Build history of the part. All positions in model axes, mm. A direction names the side the tool comes from. Give positions to 0.01 mm unless a question says otherwise; leave off trailing zeros. Order: outer loops, then holes, each group sorted by start corner. A loop starts at its lowest first (then second) coordinate and runs counter-clockwise, first axis right, second up. Notation, with made-up numbers: (73.5, -13) - (125.5, -13) arc R16 cw to (125.5, 4) - close; hole circle Ø7 at (72.5, -7.75). An arc over 180 degrees is marked (long way). Answer in a Markdown table with one row per item.
```python
from build123d import *

# Parameters (mm, degrees)
SKETCH1_R           = 0.75
SKETCH1_R_2         = 3.75
BOSS_EXTRUDE1_DEPTH = 3
SKETCH2_W           = 3
SKETCH2_H           = 20
BOSS_EXTRUDE2_DEPTH = 52.5
FILLET5_R           = 10


with BuildPart() as part:
    # Sketch1 → Boss-Extrude1 (new body)
    with BuildSketch(Plane.XY):
        Polygon((0, 0), (-10, 0), (-10, 35), (0, 35), (10, 35), (10, 0), align=None)
        with Locations((-5, 31.95)):
            Circle(SKETCH1_R, mode=Mode.SUBTRACT)
        with Locations((-5, 3.05)):
            Circle(SKETCH1_R, mode=Mode.SUBTRACT)
        with Locations((-5, 17.5)):
            Circle(SKETCH1_R_2, mode=Mode.SUBTRACT)
    extrude(amount=BOSS_EXTRUDE1_DEPTH)

    # Sketch2 → Boss-Extrude2 (add)
    with BuildSketch(Plane(origin=(0, 35, 0), x_dir=(1, 0, 0), z_dir=(0, 1, 0))):
        with Locations((8.5, -10)):
            Rectangle(SKETCH2_W, SKETCH2_H)
    extrude(amount=BOSS_EXTRUDE2_DEPTH)

    # Fillet5
    fillet5_edges = [part.edges().sort_by_distance(p)[0] for p in [
        (8.5, 35, 3),
    ]]
    fillet(fillet5_edges, radius=FILLET5_R)


solid = part.part
```
1. Cut at C-C on y = 3.05. Write the cut outline in (x, z).
Check result:
| item | result |
|---|---|
| outline | (-10, 0) - (-5.75, 0) - (-5.75, 3) - (-10, 3) - close; (-4.25, 0) - (10, 0) - (10, 3) - (-4.25, 3) - close |
2. Two-plate mould, pull along Y, no slides. Class faces 4 (the face through (8, 61, 20)), 5 (the face through (8.48, 31.99, 5.85)), 6 (the face through (-5.098, 32.694, 1.479)): +Y half, -Y half, draft (parallel to the pull), parting line (faces both ways), or undercut.
Check result:
| item | result |
|---|---|
| face 4 | draft |
| face 5 | -Y half |
| face 6 | undercut |
3. Probe line 1 (Y direction, x = -5, z = 2.3); line 2 (Z direction, x = 0, y = 34.5); line 3 (X direction, y = 49, z = 13.75). List the from-to ranges inside material, lowest first.
Check result:
| item | result |
|---|---|
| line 1 | y = 0 to 2.3, 3.8 to 13.75, 21.25 to 31.2, 32.7 to 35 |
| line 2 | z = 0 to 3 |
| line 3 | x = 7 to 10 |
4. Cut at A-A on x = -5. Write the cut outline in (y, z), and give its area (3 significant figures).
Check result:
| item | result |
|---|---|
| outline | (0, 0) - (2.3, 0) - (2.3, 3) - (0, 3) - close; (3.8, 0) - (13.75, 0) - (13.75, 3) - (3.8, 3) - close; (21.25, 0) - (31.2, 0) - (31.2, 3) - (21.25, 3) - close; (32.7, 0) - (35, 0) - (35, 3) - (32.7, 3) - close |
| area | 73.5 mm² |
5. Which spindle directions (+Z, -Z, +X, -X, +Y, -Y) get a long thin tool onto all of the face, cutting with end or side? Do faces 1 (the face through (0, 0, 1)), 2 (the face through (8, 35, 16)), 3 (the face through (-1, 35, 1)). Say none if no direction does.
Check result:
| item | result |
|---|---|
| face 1 | +Z, -Z, +X, -X, -Y |
| face 2 | +Z, +X, -X, -Y |
| face 3 | +Z, -Z, -X, +Y |
6. Drop flat-ended pins along their axis: P1, Ø8, axis at y = 57.5, z = 10, coming from the -X side; P2, Ø3.5, axis at x = -2.5, z = 1.5, coming from the +Y side; P3, Ø0.9, axis at x = 8.5, z = 17, coming from the -Y side. Give the stop position or say it passes through.
Check result:
| item | result |
|---|---|
| P1 | stops at x = 7 |
| P2 | stops at y = 35 |
| P3 | stops at y = 35 |
7. Cut at D-D on z = 10.5. Write the cut outline in (x, y), and give its area (3 significant figures).
Check result:
| item | result |
|---|---|
| outline | (7, 34.68) - (10, 34.68) - (10, 87.5) - (7, 87.5) - close |
| area | 158 mm² |
8. Cut at B-B on y = 17.5. Write the cut outline in (x, z).
Check result:
| item | result |
|---|---|
| outline | (-10, 0) - (-8.75, 0) - (-8.75, 3) - (-10, 3) - close; (-1.25, 0) - (10, 0) - (10, 3) - (-1.25, 3) - close |
